The listing builds one solid part. Answer for the finished solid, in the listing's coordinates (mm). Coordinates: 2 decimals unless noted, no trailing zeros. Loops run counter-clockwise (first coordinate to the right, second up) from the corner with the lowest first, then second, coordinate; pieces in that order, holes last. Notation, with made-up numbers: (-34.5, -37.5) - (20.5, -37.5) arc R18 cw to (20.5, -26.5) - close; hole circle Ø6 at (79.25, 13). An arc over 180 degrees is marked (long way). One line per question, with ' | ' between items.
from build123d import *

# Parameters (mm, degrees)
SKETCH1_R               = 14.2875
BOSS_EXTRUDE1_DEPTH     = 25.4
SKETCH2_R               = 3.302
CUT_EXTRUDE1_DEPTH      = 8
CUT_EXTRUDE2_DEPTH      = 33.456514177
CUT_EXTRUDE2_DEPTH_BACK = 33.456514177
SKETCH3_R               = 2.4765
CHAMFER1_SIZE           = 2.54
CUT_EXTRUDE3_DEPTH      = 33.456514265
CUT_EXTRUDE3_DEPTH_BACK = 33.456514265
SKETCH4_R               = 2.413


with BuildPart() as part:
    # Sketch1 → Boss-Extrude1 (new body)
    with BuildSketch(Plane(origin=(0, 0, 0), x_dir=(1, 0, 0), z_dir=(0, 1, 0))):
        with Locations(Location((0, 0, 0), (0, 0, 270))):
            Circle(SKETCH1_R)
    extrude(amount=BOSS_EXTRUDE1_DEPTH)

    # Sketch2 → Cut-Extrude1 (cut)
    with BuildSketch(Plane(origin=(0, 0, 0), x_dir=(-1, 0, 0), z_dir=(0, -1, 0))):
        with Locations(Location((0, 0, 0), (0, 0, 90))):
            Circle(SKETCH2_R)
    extrude(amount=-CUT_EXTRUDE1_DEPTH, mode=Mode.SUBTRACT)

    # Sketch3 → Cut-Extrude2 (cut, two sides: drawn at the far end of the back side and taken through both)
    with BuildSketch(Plane(origin=(0, 0, 0), x_dir=(0, 0, -1), z_dir=(1, 0, 0)).offset(-CUT_EXTRUDE2_DEPTH_BACK)):
        with Locations((0, 12.7)):
            Circle(SKETCH3_R)
    extrude(amount=CUT_EXTRUDE2_DEPTH + CUT_EXTRUDE2_DEPTH_BACK, mode=Mode.SUBTRACT)

    # Chamfer1
    chamfer1_edges = [part.edges().sort_by_distance(p)[0] for p in [
        (0, 25.4, -14.2875),
    ]]
    chamfer(chamfer1_edges, length=CHAMFER1_SIZE)

    # Sketch4 → Cut-Extrude3 (cut, two sides: drawn at the far end of the back side and taken through both)
    with BuildSketch(Plane.XY.offset(-CUT_EXTRUDE3_DEPTH_BACK)):
        with Locations((0, 12.7)):
            Circle(SKETCH4_R)
    extrude(amount=CUT_EXTRUDE3_DEPTH + CUT_EXTRUDE3_DEPTH_BACK, mode=Mode.SUBTRACT)


solid = part.part
Item 1: Each of these flat-tipped pins is pushed along its axis until it touches: pin 1 Ø8 at (x, y) = (-5.5, 5) entering from -Z; pin 2 Ø1 at (y, z) = (12.5, 6) entering from -X; pin 3 Ø4.5 at (x, y) = (0, 12.7) entering from -Z; pin 4 Ø10 at (x, y) = (-11, 9) entering from +Z. Where does it stop, or does it pass through?
Taken from the geometry:
pin 1: stops at z = -14.21 | pin 2: stops at x = -13.19 | pin 3: passes through | pin 4: stops at z = 12.97
Item 2: Find section C-C, the plane y = 10.75. Write down the section's boundary in (x, z) (1 decimal).
Taken from the geometry:
outline: (-14.2, -1.5) arc R14.3 ccw to (-1.4, -14.2) - (-1.4, -1.5) - close; (-14.2, 1.5) - (-1.4, 1.5) - (-1.4, 14.2) arc R14.3 ccw to start; (1.4, -14.2) arc R14.3 ccw to (14.2, -1.5) - (1.4, -1.5) - close; (1.4, 1.5) - (14.2, 1.5) arc R14.3 ccw to (1.4, 14.2) - close
Item 3: Find the intervals of material crossed by line 1 (Y direction, x = 0.25, z = 0); line 2 (Y direction, x = 3.75, z = 0); line 3 (Z direction, x = -0.5, y = 18.5), in increasing order. Write a range as [from, to].
Taken from the geometry:
line 1: y = [8, 10.22], [15.18, 25.4] | line 2: y = [0, 10.22], [15.18, 25.4] | line 3: z = [-14.28, 14.28]
Item 4: Find section A-A, the plane z = 0. Write down the section's boundary in (x, y).
Taken from the geometry:
outline: (-14.29, 0) - (-3.3, 0) - (-3.3, 8) - (3.3, 8) - (3.3, 0) - (14.29, 0) - (14.29, 10.22) - (-14.29, 10.22) - close; (-14.29, 15.18) - (14.29, 15.18) - (14.29, 22.86) - (11.75, 25.4) - (-11.75, 25.4) - (-14.29, 22.86) - close
Item 5: Find section B-B, the plane x = 0. Write down the section's boundary in (y, z).
Taken from the geometry:
outline: (0, -14.29) - (10.29, -14.29) - (10.29, -0.56) arc R2.48 cw to (10.29, 0.56) - (10.29, 14.29) - (0, 14.29) - (0, 3.3) - (8, 3.3) - (8, -3.3) - (0, -3.3) - close; (15.11, -14.29) - (22.86, -14.29) - (25.4, -11.75) - (25.4, 11.75) - (22.86, 14.29) - (15.11, 14.29) - (15.11, 0.56) arc R2.48 cw to (15.11, -0.56) - close
Item 6: Find section D-D, the plane y = 6.5. Write down the section's boundary in (x, z) (1 decimal).
Taken from the geometry:
outline: circle Ø28.6 at (0, 0); hole circle Ø6.6 at (0, 0)
Item 7: The mould has two halves that part along Z. Classify faces 1 (the face through (-10.531, 25.277, 5.478)), 2 (the face through (-2.41, 12.81, 7.33)), 3 (the face through (0.99, 3.94, -3.15)), 4 (the face through (0, 8, 0)): pulls with the +Z half, pulls with the -Z half, needs draft (parallel to the pull), parting line crosses it, or undercut.
Taken from the geometry:
face 1: parting line crosses it | face 2: needs draft | face 3: undercut | face 4: undercut
